```python
from build123d import *

# Parameters (mm, degrees)
F0_R     = 10
F1_DEPTH = 25
F2_T     = -1
F3_R     = 1


with BuildPart() as f1:
    # F0 (on Top) → F1 (new body)
    with BuildSketch(Plane.XY):
        Circle(F0_R)
    extrude(amount=F1_DEPTH)

    # F2
    f2_openings = [f1.faces().sort_by_distance(p)[0] for p in [
        (0, 0, 0),
    ]]
    offset(amount=F2_T, openings=f2_openings)

    # F3
    f3_edges = [f1.edges().sort_by_distance(p)[0] for p in [
        (-10, 0, 25),
    ]]
    fillet(f3_edges, radius=F3_R)


solid = f1.part
```
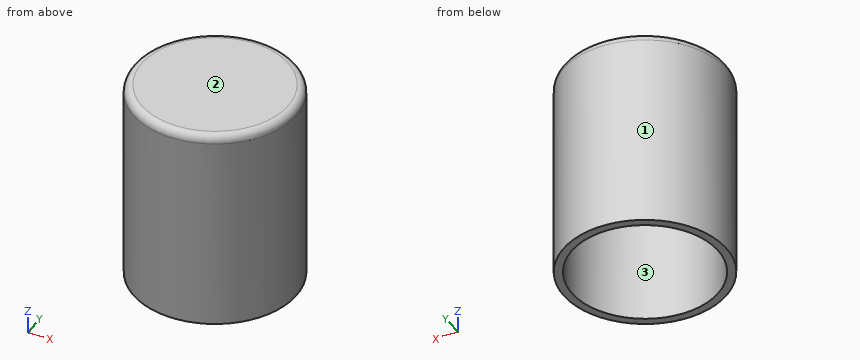
For this review, take the finished solid that the model builds, in its own axes (mm). Face numbers are marked on the shaded views. Round coordinates to 2 decimals unless told otherwise and drop trailing zeros. Write each loop counter-clockwise with the first axis right and the second up, starting at its lowest first coordinate (ties: lowest second). Pieces come first, ordered by that corner, then holes. Notation, with made-up numbers: (40.25, -38) - (84.25, -38) arc R35 ccw to (84.25, 1) - close; hole circle Ø3 at (21.5, 48). An arc over 180 degrees is marked (long way). Answer as a JSON object with one key per item and string values.
1. We need section B-B on z = 16. Give the boundary of the cut face in (x, y), then the cut area to 3 significant figures.
Response values:
{"outline": "circle Ø20 at (0, 0); hole circle Ø18 at (0, 0)", "area": "59.7 mm2"}
2. We need section A-A on x = 0. Give the boundary of the cut face in (y, z).
Response values:
{"outline": "(-10, 0) - (-9, 0) - (-9, 24) - (9, 24) - (9, 0) - (10, 0) - (10, 24) arc R1 ccw to (9, 25) - (-9, 25) arc R1 ccw to (-10, 24) - close"}
3. For pin 1 Ø10 at (y, z) = (7, 14.5) entering from -X; pin 2 Ø12 at (y, z) = (-6.5, 4.5) entering from +X; pin 3 Ø6 at (x, z) = (3.5, 7.5) entering from -Y, all flat-tipped, find the tip position at first contact; note any pin that passes through.
Response values:
{"pin 1": "stops at x = -9.8", "pin 2": "stops at x = 9.99", "pin 3": "stops at y = -9.99"}
4. To check wall thickness, follow line 1 along Y through (x, z) = (0, 14.5); line 2 along Z through (x, y) = (5.5, 5.25); line 3 along X through (y, z) = (-4.25, 18). State the ranges of each line that lie inside material, in increasing order.
Response values:
{"line 1": "y = -10 to -9, 9 to 10", "line 2": "z = 24 to 25", "line 3": "x = -9.05 to -7.93, 7.93 to 9.05"}
5. Draft analysis for pull direction Y (two halves, no side actions). For the marked faces 1, 2 and 3, state which applies: +Y half, -Y half, draft (parallel to the pull), parting line (faces both ways), or undercut.
Response values:
{"face 1": "parting line", "face 2": "draft", "face 3": "undercut"}
